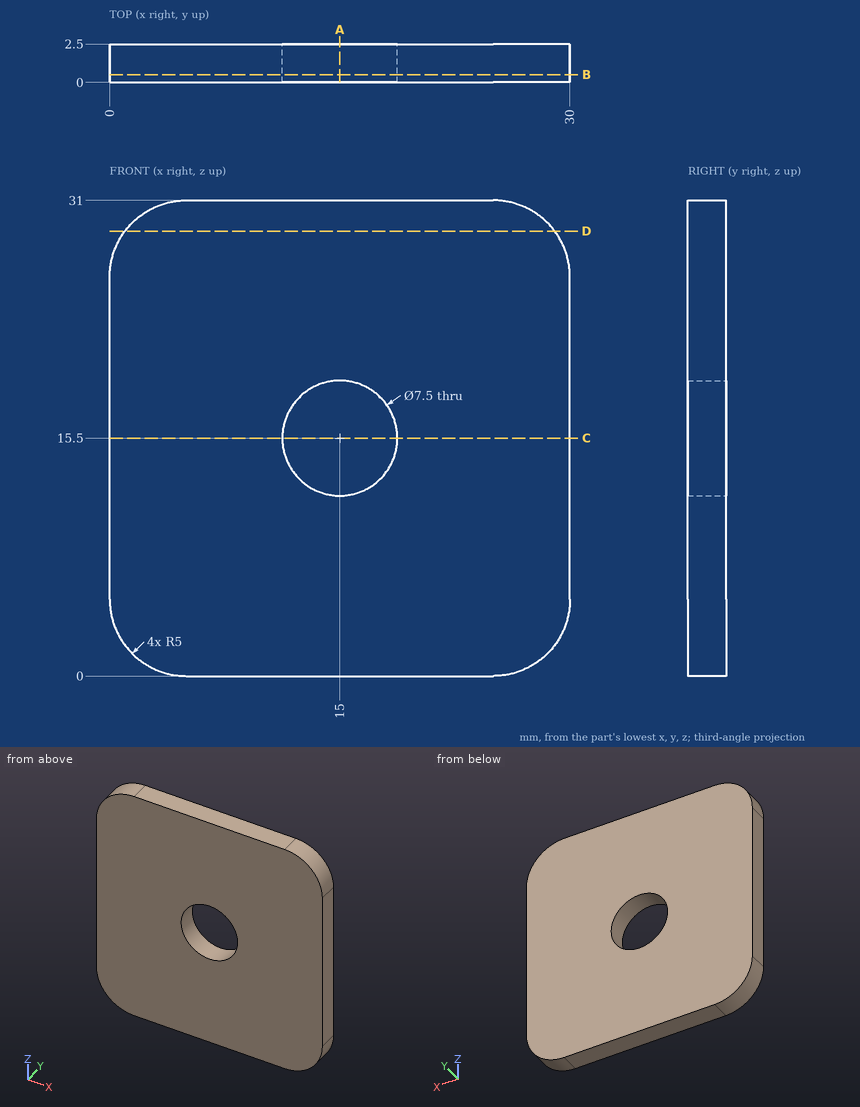
Source: three-view drawing plus pictorial views. Frame: mm from the lowest corner of the part. Round coordinates to 2 decimals unless told otherwise and drop trailing zeros. Write each loop counter-clockwise with the first axis right and the second up, starting at its lowest first coordinate (ties: lowest second). Pieces come first, ordered by that corner, then holes. Notation, with made-up numbers: M 27.5,82 L 79.5,82 A14 cw 79.5,102 Z; hole C -18,-25 d1. An arc over 180 degrees is marked long. Write each question's results on one line, items separated by ' | '.
Q1. Section query D-D (z = 29). Return loops of the section in (x, y).
Results:
outline: M 1,0 L 29,0 L 29,2.5 L 1,2.5 Z
Q2. Pin query (flat end, axial travel): P1, Ø2, axis at x = 3.5, z = 3, coming from the -Y side; P2, Ø3, axis at x = 16, z = 16.5, coming from the -Y side. Return the tip coordinate at first contact, or that it passes through.
Results:
P1: stops at y = 0 | P2: passes through
Q3. Line query: line 1 along Z through (x, y) = (15, 0.75); line 2 along Z through (x, y) = (17.75, 2.2); line 3 along X through (y, z) = (2.45, 4). Output: solid intervals per line, ascending.
Results:
line 1: z = 0 to 11.75, 19.25 to 31 | line 2: z = 0 to 12.95, 18.05 to 31 | line 3: x = 0.1 to 29.9
Q4. Section query C-C (z = 15.5). Return loops of the section in (x, y).
Results:
outline: M 0,0 L 11.25,0 L 11.25,2.5 L 0,2.5 Z; M 18.75,0 L 30,0 L 30,2.5 L 18.75,2.5 Z
Q5. Section query B-B (y = 0.5). Return loops of the section in (x, z), and give its area (3 significant figures).
Results:
outline: M 0,5 A5 ccw 5,0 L 25,0 A5 ccw 30,5 L 30,26 A5 ccw 25,31 L 5,31 A5 ccw 0,26 Z; hole C 15,15.5 d7.5 | area: 864 mm^2
Q6. Section query A-A (x = 15). Return loops of the section in (y, z).
Results:
outline: M 0,0 L 2.5,0 L 2.5,11.75 L 0,11.75 Z; M 0,19.25 L 2.5,19.25 L 2.5,31 L 0,31 Z
